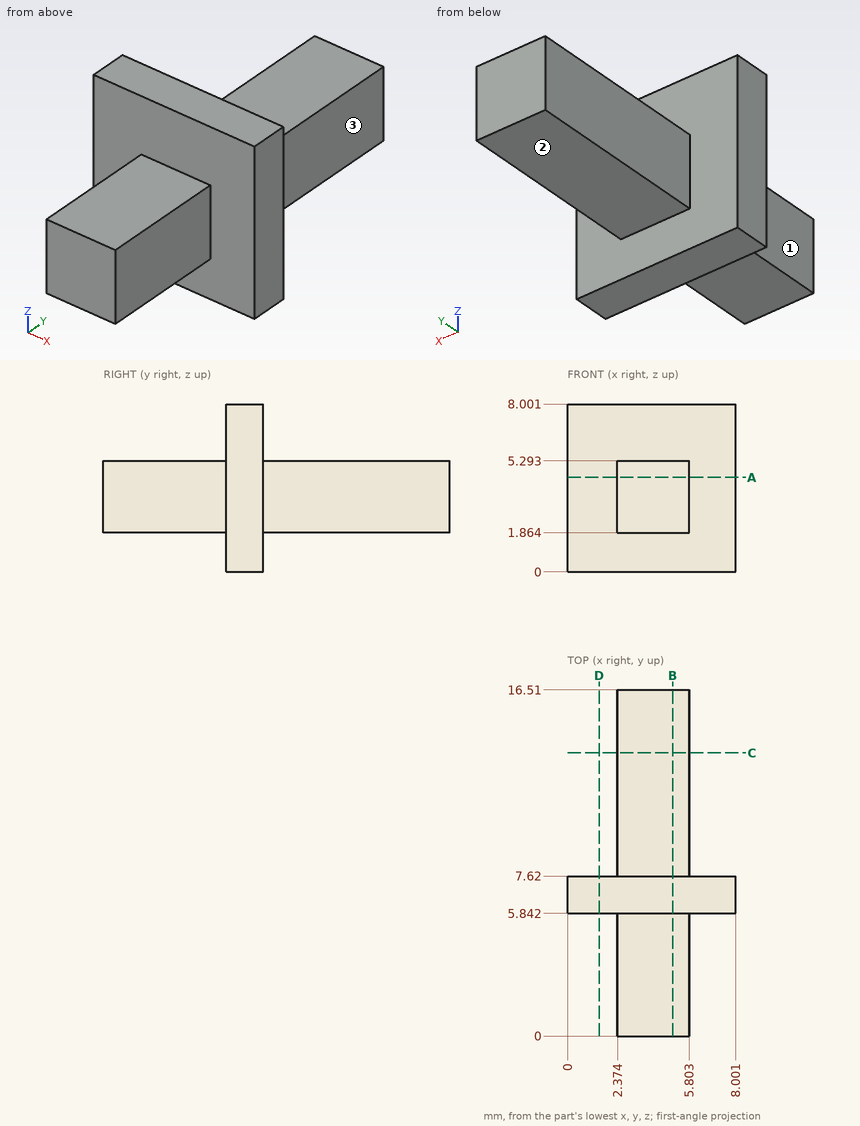
Geometry check sheet. Reference: drawing and pictorial views, mm from the part's lowest x, y, z. A direction names the side the tool comes from. Round coordinates to 2 decimals unless told otherwise and drop trailing zeros. Loops run counter-clockwise (first coordinate to the right, second up) from the corner with the lowest first, then second, coordinate; pieces in that order, holes last. Notation, with made-up numbers: M 89.25,80 L 109.25,80 A22 ccw 109.25,118 Z; hole C 26,37 d8. An arc over 180 degrees is marked long. One line per item, written item: value.
(1) Sectioned sample at C-C, the plane y = 13.5. Record the cut outline in (x, z).
Computed values:
outline: M 2.37,1.86 L 5.8,1.86 L 5.8,5.29 L 2.37,5.29 Z
(2) Access from +Z, -Z, +X, -X, +Y, -Y to the whole of each face (thin tool, end or side, straight path). Record for the marked faces 1, 2 and 3.
Computed values:
face 1: +Z, -Z, -X, -Y
face 2: -Z, +X, -X, +Y
face 3: +Z, -Z, +X, +Y
(3) Sectioned sample at A-A, the plane z = 4.5. Record the cut outline in (x, y).
Computed values:
outline: M 0,5.84 L 2.37,5.84 L 2.37,0 L 5.8,0 L 5.8,5.84 L 8,5.84 L 8,7.62 L 5.8,7.62 L 5.8,16.51 L 2.37,16.51 L 2.37,7.62 L 0,7.62 Z
(4) Thickness scan on line 1 (Y direction, x = 7.5, z = 1.5); line 2 (Z direction, x = 3.5, y = 2); line 3 (X direction, y = 4.25, z = 2.75). Record the ranges inside material, lowest first.
Computed values:
line 1: y = 5.84 to 7.62
line 2: z = 1.86 to 5.29
line 3: x = 2.37 to 5.8
(5) Depth check by flat-ended pin: pin 1 Ø1 at (x, y) = (6.5, 5.5) entering from -Z; pin 2 Ø1 at (x, z) = (5, 7) entering from +Y; pin 3 Ø2.5 at (x, y) = (5, 3.5) entering from -Z; pin 4 Ø2.5 at (y, z) = (1.5, 3.5) entering from +X. Enter the tip coordinate at first touch or a pass-through.
Computed values:
pin 1: stops at z = 0
pin 2: stops at y = 7.62
pin 3: stops at z = 1.86
pin 4: stops at x = 5.8
(6) Sectioned sample at D-D, the plane x = 1.5. Record the cut outline in (y, z).
Computed values:
outline: M 5.84,0 L 7.62,0 L 7.62,8 L 5.84,8 Z
(7) Sectioned sample at B-B, the plane x = 5. Record the cut outline in (y, z).
Computed values:
outline: M 0,1.86 L 5.84,1.86 L 5.84,0 L 7.62,0 L 7.62,1.86 L 16.51,1.86 L 16.51,5.29 L 7.62,5.29 L 7.62,8 L 5.84,8 L 5.84,5.29 L 0,5.29 Z
